from build123d import *

# Parameters (mm, degrees)
BOSS_EXTRUDE1_DEPTH     = 8
SKETCH2_R               = 2.5
CUT_EXTRUDE1_DEPTH      = 8
SKETCH3_W               = 65
SKETCH3_H               = 30
CUT_EXTRUDE2_DEPTH      = 4
MIRROR2_COPY_1_SKETCH_W = 65
MIRROR2_COPY_1_SKETCH_H = 30
MIRROR2_COPY_1_DEPTH    = 4


with BuildPart() as part:
    # Sketch1 → Boss-Extrude1 (new body)
    with BuildSketch(Plane(origin=(0, 0, 0), x_dir=(1, 0, 0), z_dir=(0, 1, 0))):
        Polygon((125, 160), (-125, 160), (-125, 120), (-165, 120), (-165, -120), (-125, -120), (-125, -160), (125, -160), (125, -120), (165, -120), (165, 120), (125, 120), align=None)
    extrude(amount=BOSS_EXTRUDE1_DEPTH)

    # Sketch2 → Cut-Extrude1 (cut)
    with BuildSketch(Plane(origin=(0, 8, 0), x_dir=(1, 0, 0), z_dir=(0, 1, 0))):
        with Locations(Location((155, 60, 0), (0, 0, 270))):
            Circle(SKETCH2_R)
        with Locations(Location((155, 0, 0), (0, 0, 270))):
            Circle(SKETCH2_R)
        with Locations(Location((155, -60, 0), (0, 0, 270))):
            Circle(SKETCH2_R)
        with Locations(Location((40, -150, 0), (0, 0, 270))):
            Circle(SKETCH2_R)
        with Locations(Location((-40, -150, 0), (0, 0, 270))):
            Circle(SKETCH2_R)
        with Locations(Location((-155, -60, 0), (0, 0, 90))):
            Circle(SKETCH2_R)
        with Locations(Location((-155, 0, 0), (0, 0, 90))):
            Circle(SKETCH2_R)
        with Locations(Location((-155, 60, 0), (0, 0, 90))):
            Circle(SKETCH2_R)
        with Locations(Location((-40, 150, 0), (0, 0, 90))):
            Circle(SKETCH2_R)
        with Locations(Location((40, 150, 0), (0, 0, 90))):
            Circle(SKETCH2_R)
    extrude(amount=-CUT_EXTRUDE1_DEPTH, mode=Mode.SUBTRACT)

    # Sketch3 → Cut-Extrude2 (cut)
    with BuildSketch(Plane(origin=(0, 8, 0), x_dir=(1, 0, 0), z_dir=(0, 1, 0))):
        with Locations((-92.5, 145)):
            Rectangle(SKETCH3_W, SKETCH3_H)
    cut_extrude2 = extrude(amount=-CUT_EXTRUDE2_DEPTH, mode=Mode.SUBTRACT)

    # Mirror1: Cut-Extrude2 across plane
    add(cut_extrude2.mirror(Plane(origin=(0, 0, 0), x_dir=(1, 0, 0), z_dir=(0, 0, -1))), mode=Mode.SUBTRACT)

    # Mirror2: Cut-Extrude2 across plane
    add(cut_extrude2.mirror(Plane.ZY), mode=Mode.SUBTRACT)

    # Mirror2 copy 1 sketch → Mirror2 copy 1 (cut)
    with BuildSketch(Plane(origin=(0, 8, 0), x_dir=(-1, 0, 0), z_dir=(0, 1, 0))):
        with Locations((-92.5, 145)):
            Rectangle(MIRROR2_COPY_1_SKETCH_W, MIRROR2_COPY_1_SKETCH_H)
    extrude(amount=-MIRROR2_COPY_1_DEPTH, mode=Mode.SUBTRACT)


solid = part.part
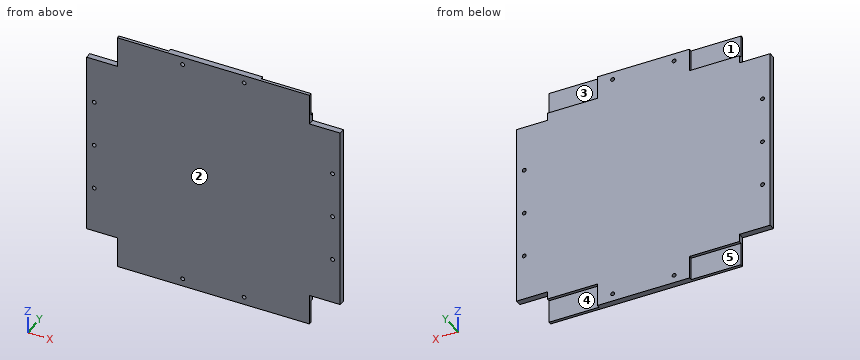
Model file for the job. Use its own axes, mm. Face numbers are marked on the shaded views. A direction names the side the tool comes from. Give positions to 0.01 mm unless a question says otherwise; leave off trailing zeros. Order: outer loops, then holes, each group sorted by start corner. A loop starts at its lowest first (then second) coordinate and runs counter-clockwise, first axis right, second up. Notation, with made-up numbers: (39.25, 14.5) - (98.25, 14.5) arc R26 ccw to (98.25, 51.5) - close; hole circle Ø5 at (56, 39.25). An arc over 180 degrees is marked (long way). One line per item, written item: value.
Item 1: Slice it at B-B (z = -137.5). List the corners of the cut face in (x, y).
Response values:
outline: (-125, 0) - (125, 0) - (125, 4) - (60, 4) - (60, 8) - (-60, 8) - (-60, 4) - (-125, 4) - close
Item 2: Tool access for the marked faces 1, 2, 3, 4 and 5: list every direction of +Z, -Z, +X, -X, +Y, -Y with a clear straight run to the whole face (end or side of a thin tool).
Response values:
face 1: +Z, -X, +Y
face 2: +Z, -Z, +X, -X, -Y
face 3: +Z, +X, +Y
face 4: -Z, +X, +Y
face 5: -Z, -X, +Y
Item 3: Wall check: line 1 (X direction, y = 2.25, z = 150); line 2 (X direction, y = 4.25, z = -150); line 3 (Z direction, x = 155, y = 3.25). Give the ranges that are in metal, low to high.
Response values:
line 1: -125 to -42.5, -37.5 to 37.5, 42.5 to 125
line 2: -60 to -42.5, -37.5 to 37.5, 42.5 to 60
line 3: -120 to -62.5, -57.5 to -2.5, 2.5 to 57.5, 62.5 to 120
Item 4: Pin check, flat tips, straight feed: pin 1 Ø3 at (x, y) = (99.5, 7) entering from +Z; pin 2 Ø2 at (x, y) = (-80, 5.5) entering from -Z; pin 3 Ø2 at (y, z) = (5.5, 151.5) entering from +X. Stop position of each tip, or through.
Response values:
pin 1: z = 130
pin 2: z = -130
pin 3: x = 60
Item 5: Slice it at A-A (x = 94). List the corners of the cut face in (y, z), then the cut area to 3 significant figures.
Response values:
outline: (0, -160) - (4, -160) - (4, -130) - (8, -130) - (8, 130) - (4, 130) - (4, 160) - (0, 160) - close
area: 2,320 mm2
Item 6: Slice it at C-C (z = 126). List the corners of the cut face in (x, y), then the cut area to 3 significant figures.
Response values:
outline: (-125, 0) - (125, 0) - (125, 8) - (-125, 8) - close
area: 2,000 mm2
